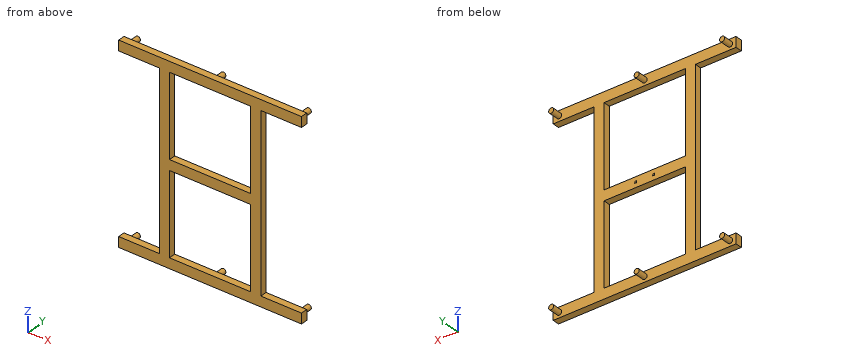
```python
from build123d import *

# Parameters (mm, degrees)
SKETCH1_W           = 300
SKETCH1_H           = 570
SKETCH1_W_2         = 240
SKETCH1_H_2         = 240
BOSS_EXTRUDE1_DEPTH = 20
SKETCH1_3_W         = 120
SKETCH1_3_H         = 30
BOSS_EXTRUDE2_DEPTH = 20
SKETCH2_R           = 7.5
BOSS_EXTRUDE3_DEPTH = 30
SKETCH4_W           = 5
SKETCH4_H           = 5
BOSS_EXTRUDE4_DEPTH = 1


with BuildPart() as part:
    # Sketch1 → Boss-Extrude1 (new body)
    with BuildSketch(Plane(origin=(0, 0, 0), x_dir=(1, 0, 0), z_dir=(0, 1, 0))):
        Rectangle(SKETCH1_W, SKETCH1_H)
        with Locations((0, 135)):
            Rectangle(SKETCH1_W_2, SKETCH1_H_2, mode=Mode.SUBTRACT)
        with Locations((0, -135)):
            Rectangle(SKETCH1_W_2, SKETCH1_H_2, mode=Mode.SUBTRACT)
    extrude(amount=BOSS_EXTRUDE1_DEPTH)

    # Sketch1_3 → Boss-Extrude2 (add)
    with BuildSketch(Plane(origin=(0, 0, 0), x_dir=(1, 0, 0), z_dir=(0, 1, 0))):
        with Locations((210, 270)):
            Rectangle(SKETCH1_3_W, SKETCH1_3_H)
        with Locations((-210, 270)):
            Rectangle(SKETCH1_3_W, SKETCH1_3_H)
        with Locations((-210, -270)):
            Rectangle(SKETCH1_3_W, SKETCH1_3_H)
        with Locations((210, -270)):
            Rectangle(SKETCH1_3_W, SKETCH1_3_H)
    extrude(amount=BOSS_EXTRUDE2_DEPTH)

    # Sketch2 → Boss-Extrude3 (add)
    with BuildSketch(Plane(origin=(0, 20, 0), x_dir=(1, 0, 0), z_dir=(0, 1, 0))):
        with Locations(Location((0, 270, 0), (0, 0, 270))):
            Circle(SKETCH2_R)
        with Locations(Location((252.5, 270, 0), (0, 0, 270))):
            Circle(SKETCH2_R)
        with Locations(Location((-252.5, 270, 0), (0, 0, 270))):
            Circle(SKETCH2_R)
        with Locations(Location((-252.5, -270, 0), (0, 0, 270))):
            Circle(SKETCH2_R)
        with Locations(Location((252.5, -270, 0), (0, 0, 270))):
            Circle(SKETCH2_R)
        with Locations(Location((0, -270, 0), (0, 0, 270))):
            Circle(SKETCH2_R)
    extrude(amount=BOSS_EXTRUDE3_DEPTH)

    # Sketch4 → Boss-Extrude4 (add)
    with BuildSketch(Plane(origin=(0, 20, 0), x_dir=(1, 0, 0), z_dir=(0, 1, 0))):
        with Locations((-26.5, 0)):
            Rectangle(SKETCH4_W, SKETCH4_H)
        with Locations((26.5, 0)):
            Rectangle(SKETCH4_W, SKETCH4_H)
    extrude(amount=BOSS_EXTRUDE4_DEPTH)


solid = part.part
```
Source: CAD feature listing. Evaluate the final solid. Frame: model axes, mm. Coordinates: 2 decimals unless noted, no trailing zeros. Loops run counter-clockwise (first coordinate to the right, second up) from the corner with the lowest first, then second, coordinate; pieces in that order, holes last. Notation, with made-up numbers: (-7.5, 53) -> (15.5, 53) arc R29 ccw to (15.5, 75) -> close; hole circle Ø2 at (12.25, 89). An arc over 180 degrees is marked (long way). One line per item, written item: value. Start each with the question number.
Q1. Section query D-D, the plane x = 0. Return the cut outline in (y, z).
Q2. Line query: line 1 along Z through (x, y) = (2.5, 15); line 2 along X through (y, z) = (19.5, -59); line 3 along Z through (x, y) = (-218, 19). Output: solid intervals per line, ascending.
Q3. Section query C-C, the plane y = 36. Return the cut outline in (x, z), and give its area (3 significant figures).
Q4. Section query B-B, the plane z = -44. Return the cut outline in (x, y).
Q5. Section query A-A, the plane x = 252.5. Return the cut outline in (y, z), and give its area (3 significant figures).
Q6. Contact query for flat-ended pins moving along their axis: P1, Ø0.5, axis at x = -27, y = 20.5, coming from the +Z side; P2, Ø3, axis at y = 17.5, z = -168.5, coming from the -X side; P3, Ø4, axis at y = 16.5, z = -10.5, coming from the +X side. Output: stop coordinate, or through.
Results:
1. outline: (0, -285) -> (20, -285) -> (20, -277.5) -> (50, -277.5) -> (50, -262.5) -> (20, -262.5) -> (20, -255) -> (0, -255) -> close; (0, -15) -> (20, -15) -> (20, 15) -> (0, 15) -> close; (0, 255) -> (20, 255) -> (20, 262.5) -> (50, 262.5) -> (50, 277.5) -> (20, 277.5) -> (20, 285) -> (0, 285) -> close
2. line 1: -285 to -255, -15 to 15, 255 to 285
2. line 2: -150 to -120, 120 to 150
2. line 3: -285 to -255, 255 to 285
3. outline: circle Ø15 at (-252.5, -270); circle Ø15 at (-252.5, 270); circle Ø15 at (0, -270); circle Ø15 at (0, 270); circle Ø15 at (252.5, -270); circle Ø15 at (252.5, 270)
3. area: 1,060 mm^2
4. outline: (-150, 0) -> (-120, 0) -> (-120, 20) -> (-150, 20) -> close; (120, 0) -> (150, 0) -> (150, 20) -> (120, 20) -> close
5. outline: (0, -285) -> (20, -285) -> (20, -277.5) -> (50, -277.5) -> (50, -262.5) -> (20, -262.5) -> (20, -255) -> (0, -255) -> close; (0, 255) -> (20, 255) -> (20, 262.5) -> (50, 262.5) -> (50, 277.5) -> (20, 277.5) -> (20, 285) -> (0, 285) -> close
5. area: 2,100 mm^2
6. P1: z = 2.5
6. P2: x = -150
6. P3: x = 150
